Geometry check sheet. Reference: the model listing, model coordinates, mm. Give positions to 0.01 mm unless a question says otherwise; leave off trailing zeros. Loops run counter-clockwise (first coordinate to the right, second up) from the corner with the lowest first, then second, coordinate; pieces in that order, holes last. Notation, with made-up numbers: (46.25, -6) -> (72.25, -6) arc R29 ccw to (72.25, 17) -> close; hole circle Ø4 at (74, -13). An arc over 180 degrees is marked (long way). Answer as a JSON object with one key per item and string values.
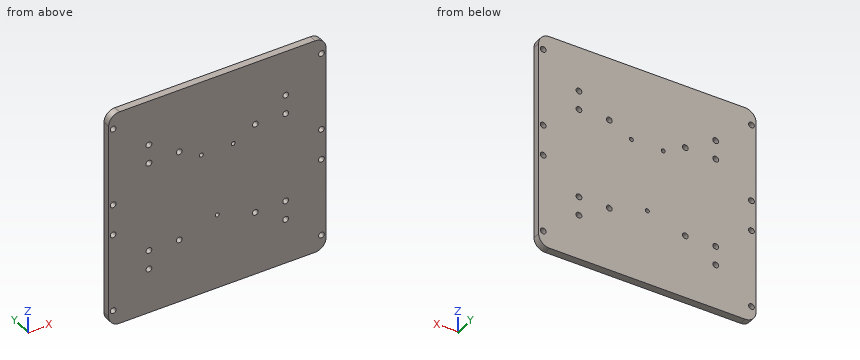
from build123d import *

# Parameters (mm, degrees)
SKETCH_1_R      = 1.6
SKETCH_1_R_2    = 1.1
EXTRUDE_1_DEPTH = 4


with BuildPart() as part:
    # 草图1 → 凸台-拉伸1 (new body)
    with BuildSketch(Plane(origin=(0, 0, 0), x_dir=(1, 0, 0), z_dir=(0, 1, 0))):
        with BuildLine():
            Line((-54, 60), (54, 60))
            ThreePointArc((54, 60), (58.242640687, 58.242640687), (60, 54))
            Line((60, 54), (60, -54))
            ThreePointArc((60, -54), (58.242640687, -58.242640687), (54, -60))
            Line((54, -60), (-54, -60))
            ThreePointArc((-54, -60), (-58.242640687, -58.242640687), (-60, -54))
            Line((-60, -54), (-60, 54))
            ThreePointArc((-60, 54), (-58.242640687, 58.242640687), (-54, 60))
        make_face()
        with Locations(Location((-57.5, 51.5, 0), (0, 0, 270))):
            Circle(SKETCH_1_R, mode=Mode.SUBTRACT)
        with Locations(Location((-57.5, 8.5, 0), (0, 0, 90))):
            Circle(SKETCH_1_R, mode=Mode.SUBTRACT)
        with Locations(Location((-37.75, 35.23, 0), (0, 0, 270))):
            Circle(SKETCH_1_R, mode=Mode.SUBTRACT)
        with Locations(Location((-37.75, 24.77, 0), (0, 0, 90))):
            Circle(SKETCH_1_R, mode=Mode.SUBTRACT)
        with Locations(Location((-57.5, -8.5, 0), (0, 0, 270))):
            Circle(SKETCH_1_R, mode=Mode.SUBTRACT)
        with Locations(Location((-37.75, -24.77, 0), (0, 0, 270))):
            Circle(SKETCH_1_R, mode=Mode.SUBTRACT)
        with Locations(Location((-37.75, -35.23, 0), (0, 0, 90))):
            Circle(SKETCH_1_R, mode=Mode.SUBTRACT)
        with Locations(Location((-57.5, -51.5, 0), (0, 0, 90))):
            Circle(SKETCH_1_R, mode=Mode.SUBTRACT)
        with Locations(Location((57.5, -51.5, 0), (0, 0, 270))):
            Circle(SKETCH_1_R, mode=Mode.SUBTRACT)
        with Locations(Location((37.75, -35.23, 0), (0, 0, 270))):
            Circle(SKETCH_1_R, mode=Mode.SUBTRACT)
        with Locations(Location((37.75, -24.77, 0), (0, 0, 90))):
            Circle(SKETCH_1_R, mode=Mode.SUBTRACT)
        with Locations(Location((57.5, -8.5, 0), (0, 0, 90))):
            Circle(SKETCH_1_R, mode=Mode.SUBTRACT)
        with Locations(Location((57.5, 8.5, 0), (0, 0, 270))):
            Circle(SKETCH_1_R, mode=Mode.SUBTRACT)
        with Locations(Location((37.75, 24.77, 0), (0, 0, 270))):
            Circle(SKETCH_1_R, mode=Mode.SUBTRACT)
        with Locations(Location((37.75, 35.23, 0), (0, 0, 90))):
            Circle(SKETCH_1_R, mode=Mode.SUBTRACT)
        with Locations(Location((57.5, 51.5, 0), (0, 0, 90))):
            Circle(SKETCH_1_R, mode=Mode.SUBTRACT)
        with Locations(Location((0, 18.6, 0), (0, 0, 270))):
            Circle(SKETCH_1_R_2, mode=Mode.SUBTRACT)
        with Locations(Location((8.8, -18.6, 0), (0, 0, 270))):
            Circle(SKETCH_1_R_2, mode=Mode.SUBTRACT)
        with Locations(Location((-8.8, -18.6, 0), (0, 0, 270))):
            Circle(SKETCH_1_R_2, mode=Mode.SUBTRACT)
        with Locations(Location((-21, 25, 0), (0, 0, 270))):
            Circle(SKETCH_1_R, mode=Mode.SUBTRACT)
        with Locations(Location((21, 25, 0), (0, 0, 90))):
            Circle(SKETCH_1_R, mode=Mode.SUBTRACT)
        with Locations(Location((21, -25, 0), (0, 0, 270))):
            Circle(SKETCH_1_R, mode=Mode.SUBTRACT)
        with Locations(Location((-21, -25, 0), (0, 0, 90))):
            Circle(SKETCH_1_R, mode=Mode.SUBTRACT)
    extrude(amount=EXTRUDE_1_DEPTH)


solid = part.part
1) Material ranges on line 1 along X through (y, z) = (2.35, 51.5); line 2 along X through (y, z) = (2, 35.23), recorded low to high. Write a range as from..to.
Geometry check:
{"line 1": "x = -60..-59.1, -55.9..55.9, 59.1..60", "line 2": "x = -60..-39.35, -36.15..36.15, 39.35..60"}
2) Section check A-A on x = 37.75. Record the cut outline in (y, z), plus the area to 3 significant figures.
Geometry check:
{"outline": "(0, -60) -> (4, -60) -> (4, -36.83) -> (0, -36.83) -> close; (0, -33.63) -> (4, -33.63) -> (4, -26.37) -> (0, -26.37) -> close; (0, -23.17) -> (4, -23.17) -> (4, 23.17) -> (0, 23.17) -> close; (0, 26.37) -> (4, 26.37) -> (4, 33.63) -> (0, 33.63) -> close; (0, 36.83) -> (4, 36.83) -> (4, 60) -> (0, 60) -> close", "area": "429 mm2"}
3) Section check C-C on z = 25. Record the cut outline in (x, y).
Geometry check:
{"outline": "(-60, 0) -> (-39.33, 0) -> (-39.33, 4) -> (-60, 4) -> close; (-36.17, 0) -> (-22.6, 0) -> (-22.6, 4) -> (-36.17, 4) -> close; (-19.4, 0) -> (19.4, 0) -> (19.4, 4) -> (-19.4, 4) -> close; (22.6, 0) -> (36.17, 0) -> (36.17, 4) -> (22.6, 4) -> close; (39.33, 0) -> (60, 0) -> (60, 4) -> (39.33, 4) -> close"}
4) Section check B-B on z = 51.5. Record the cut outline in (x, y).
Geometry check:
{"outline": "(-60, 0) -> (-59.1, 0) -> (-59.1, 4) -> (-60, 4) -> close; (-55.9, 0) -> (55.9, 0) -> (55.9, 4) -> (-55.9, 4) -> close; (59.1, 0) -> (60, 0) -> (60, 4) -> (59.1, 4) -> close"}
